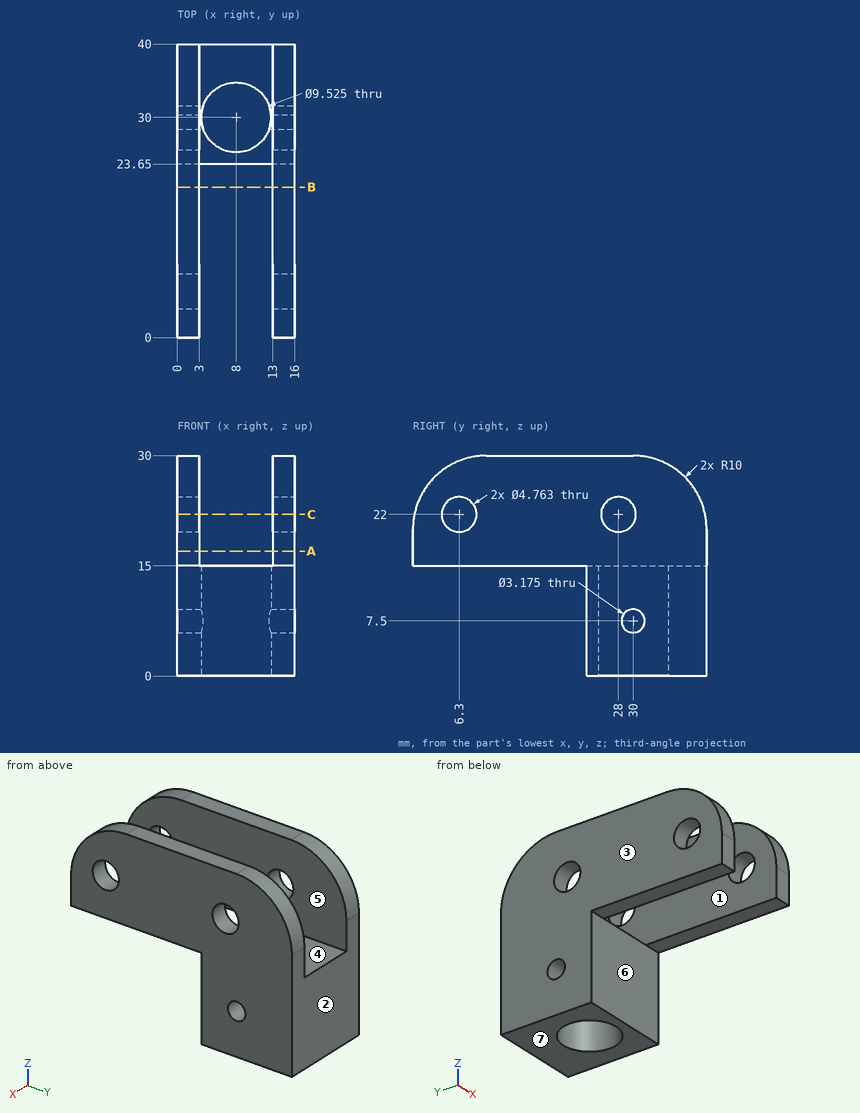
Can you work these out from the drawing? Everything is in mm from the part's minimum corner. A direction names the side the tool comes from. Coordinates: 2 decimals unless noted, no trailing zeros. Loops run counter-clockwise (first coordinate to the right, second up) from the corner with the lowest first, then second, coordinate; pieces in that order, holes last. Notation, with made-up numbers: (60.25, 6) - (114.25, 6) arc R32 ccw to (114.25, 45) - close; hole circle Ø8 at (42.5, 74). An arc over 180 degrees is marked (long way). Answer as CSV lines item,"result".
Q1. We'd pull the mould along X, two halves only. Please class the marked faces 1, 2, 3 and 4: pulls with the +X half, pulls with the -X half, needs draft (parallel to the pull), parting line crosses it, or undercut.
Response:
face 1,"undercut"
face 2,"needs draft"
face 3,"pulls with the -X half"
face 4,"undercut"
Q2. If we section it at A-A, the plane z = 17: Write out the boundary of the cut face in (x, y).
Response:
outline,"(0, 0) - (3, 0) - (3, 40) - (0, 40) - close; (13, 0) - (16, 0) - (16, 40) - (13, 40) - close"
Q3. For the marked faces 5, 6 and 7, which set-ups out of +Z, -Z, +X, -X, +Y, -Y let a thin tool reach every point of the face, with its end or its side?
Response:
face 5,"+Z, +Y, -Y"
face 6,"-Z, +X, -X, -Y"
face 7,"-Z, +X, -X, +Y, -Y"
Q4. For pin 1 (1.5 mm diameter, centred on x = 14.5, y = 17, fed in from -Z); pin 2 (4.5 mm diameter, centred on y = 28, z = 22, fed in from +X); pin 3 (2 mm diameter, centred on x = 9.5, z = 11, fed in from -Y), each with a flat end and sliding along its axis, tell me the tip position at first contact or that it passes through.
Response:
pin 1,"z = 15"
pin 2,"through"
pin 3,"y = 23.65"
Q5. If we section it at C-C, the plane z = 22: Write out the boundary of the cut face in (x, y).
Response:
outline,"(0, 0.2) - (3, 0.2) - (3, 3.92) - (0, 3.92) - close; (0, 8.68) - (3, 8.68) - (3, 25.62) - (0, 25.62) - close; (0, 30.38) - (3, 30.38) - (3, 39.8) - (0, 39.8) - close; (13, 0.2) - (16, 0.2) - (16, 3.92) - (13, 3.92) - close; (13, 8.68) - (16, 8.68) - (16, 25.62) - (13, 25.62) - close; (13, 30.38) - (16, 30.38) - (16, 39.8) - (13, 39.8) - close"
Q6. If I drill on L1, parallel to Y at x = 8, z = 7; L2, parallel to X at y = 32.5, z = 24; L3, parallel to Y at x = 15.25, z = 23, over which ranges is the centre line in solid material (lowest first)? Write a range as [from, to].
Response:
L1,"[23.65, 25.24], [34.76, 40]"
L2,"[0, 3], [13, 16]"
L3,"[0.46, 4.14], [8.46, 25.84], [30.16, 39.54]"
Q7. If we section it at B-B, the plane y = 20.5: Write out the boundary of the cut face in (x, z).
Response:
outline,"(0, 15) - (3, 15) - (3, 30) - (0, 30) - close; (13, 15) - (16, 15) - (16, 30) - (13, 30) - close"
